Build history of the part. All positions in model axes, mm. Face numbers are marked on the shaded views. Round coordinates to 2 decimals unless told otherwise and drop trailing zeros. Write each loop counter-clockwise with the first axis right and the second up, starting at its lowest first coordinate (ties: lowest second). Pieces come first, ordered by that corner, then holes. Notation, with made-up numbers: (41.5, -34.5) -> (90.5, -34.5) arc R34 cw to (90.5, -0.5) -> close; hole circle Ø10 at (-27.5, 72.5). An arc over 180 degrees is marked (long way). Answer in a Markdown table with one row per item. Add a question column.
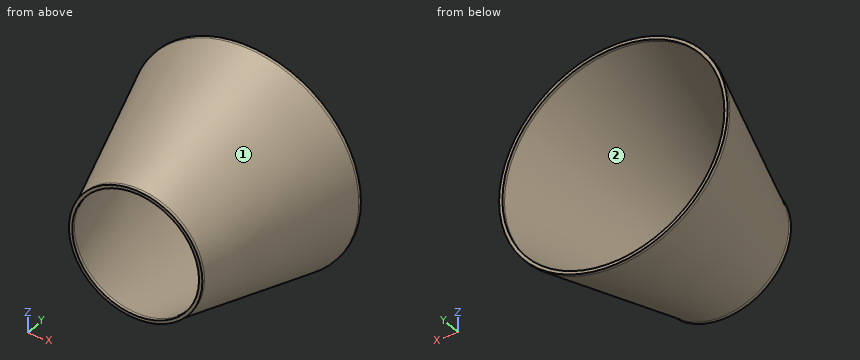
from build123d import *

# Parameters (mm, degrees)
SKETCH2_R           = 42.088061302
SKETCH2_R_2         = 40
BOSS_EXTRUDE1_DEPTH = 2
SKETCH3_R           = 72.088061302
SKETCH3_R_2         = 70
BOSS_EXTRUDE2_DEPTH = 2


with BuildPart() as part:
    # Sketch1 → Revolve1 (revolve)
    with BuildSketch(Plane.XY):
        Polygon((-40, 0), (-70, 100), (-72.088061302, 100), (-42.088061302, 0), align=None)
    revolve(axis=Axis((0, 0, 0), (0, 1, 0)))

    # Sketch2 → Boss-Extrude1 (add)
    with BuildSketch(Plane.XZ):
        Circle(SKETCH2_R)
        Circle(SKETCH2_R_2, mode=Mode.SUBTRACT)
    extrude(amount=BOSS_EXTRUDE1_DEPTH)

    # Sketch3 → Boss-Extrude2 (add)
    with BuildSketch(Plane(origin=(0, 100, 0), x_dir=(1, 0, 0), z_dir=(0, 1, 0))):
        Circle(SKETCH3_R)
        Circle(SKETCH3_R_2, mode=Mode.SUBTRACT)
    extrude(amount=BOSS_EXTRUDE2_DEPTH)


solid = part.part
(1) Saw through at D-D (y = 62). List the corners of the cut face in (x, z), plus the area to 3 significant figures.
(2) Mould opens along X. For the marked faces 1 and 2 say: pulls with the +X half, pulls with the -X half, needs draft (parallel to the pull), parting line crosses it, or undercut.
(3) Drop flat-ended pins along their axis: P1, Ø6, axis at x = 52, y = 87.5, coming from the -Z side; P2, Ø1, axis at x = -10.5, y = 42.5, coming from the +Z side; P3, Ø8, axis at y = 32.5, z = 10.5, coming from the -X side. Give the stop position or say it passes through.
(4) Saw through at B-B (x = 0). List the corners of the cut face in (y, z).
(5) Saw through at C-C (y = 83.5). List the corners of the cut face in (x, z).
(6) Saw through at A-A (z = 0). List the corners of the cut face in (x, y).
(7) Probe line 1 along X through (y, z) = (-1.5, 0); line 2 along Z through (x, y) = (0, 101). List the from-to ranges inside material, lowest first.
Answer sheet:
| question | item | result |
|---|---|---|
| 1 | outline | circle Ø121.38 at (0, 0); hole circle Ø117.2 at (0, 0) |
| 1 | area | 783 mm² |
| 2 | face 1 | parting line crosses it |
| 2 | face 2 | undercut |
| 3 | P1 | stops at z = -47.89 |
| 3 | P2 | stops at z = 54 |
| 3 | P3 | stops at x = -52.19 |
| 4 | outline | (-2, -42.09) -> (0, -42.09) -> (100, -72.09) -> (102, -72.09) -> (102, -70) -> (100, -70) -> (0, -40) -> (-2, -40) -> close; (-2, 40) -> (0, 40) -> (100, 70) -> (102, 70) -> (102, 72.09) -> (100, 72.09) -> (0, 42.09) -> (-2, 42.09) -> close |
| 5 | outline | circle Ø134.28 at (0, 0); hole circle Ø130.1 at (0, 0) |
| 6 | outline | (-72.09, 100) -> (-42.09, 0) -> (-42.09, -2) -> (-40, -2) -> (-40, 0) -> (-70, 100) -> (-70, 102) -> (-72.09, 102) -> close; (40, -2) -> (42.09, -2) -> (42.09, 0) -> (72.09, 100) -> (72.09, 102) -> (70, 102) -> (70, 100) -> (40, 0) -> close |
| 7 | line 1 | x = -42.09 to -40, 40 to 42.09 |
| 7 | line 2 | z = -72.09 to -70, 70 to 72.09 |
